Here's how the part is built. I have some questions about the finished solid (model axes, mm). Face numbers are marked on the shaded views. A direction names the side the tool comes from. Coordinates: 2 decimals unless noted, no trailing zeros. Write each loop counter-clockwise with the first axis right and the second up, starting at its lowest first coordinate (ties: lowest second). Pieces come first, ordered by that corner, then holes.
Item 1: If we section it at C-C (x = -3): Please give me the cut outline in (y, z).
Item 2: If we section it at A-A (z = 31.2): Please give me the cut outline in (x, y), then the cut area to 3 significant figures.
Item 3: If I drill on line 1 (X direction, y = 4, z = 31.2); line 2 (X direction, y = 5.75, z = 21), over which ranges is the centre line in solid material (lowest first)?
Item 4: For the marked faces 5 and 6, which set-ups out of +Z, -Z, +X, -X, +Y, -Y let a thin tool reach every point of the face, with its end or its side?
Item 5: If we section it at D-D (y = 8): Please give me the cut outline in (x, z).
Item 6: We'd pull the mould along X, two halves only. Please class the marked faces 1, 2, 3 and 4: +X half, -X half, draft (parallel to the pull), parting line (faces both ways), or undercut.
Item 7: If we section it at B-B (z = -14): Please give me the cut outline in (x, y), then the cut area to 3 significant figures.
Autodesk Inventor part; units mm, degrees
ref_plane "YZ Plane" through (0, 0, 0) normal (1, 0, 0) x (0, 1, 0)
ref_plane "XZ Plane" through (0, 0, 0) normal (0, 1, 0) x (-1, 0, 0)
ref_plane "XY Plane" through (0, 0, 0) normal (0, 0, 1) x (1, 0, 0)
sketch "Boceto1" plane through (0, 0, 0) normal (0, 1, 0) x (-1, 0, 0)
  line L0 (-41.2, 41.2) -> (41.2, 41.2)
  line L1 (41.2, 41.2) -> (41.2, -41.2)
  line L2 (41.2, -41.2) -> (-41.2, -41.2)
  line L3 (-41.2, -41.2) -> (-41.2, 41.2)
  line L4 (-41.2, 41.2) -> (41.2, -41.2) construction
  line L5 (41.2, 41.2) -> (-41.2, -41.2) construction
  line L6 (-21.2, 21.2) -> (21.2, 21.2)
  line L7 (21.2, 21.2) -> (21.2, -21.2)
  line L8 (21.2, -21.2) -> (-21.2, -21.2)
  line L9 (-21.2, -21.2) -> (-21.2, 21.2)
  line L10 (-21.2, 21.2) -> (21.2, -21.2) construction
  line L11 (21.2, 21.2) -> (-21.2, -21.2) construction
  point P0 (0, 0)
  dimension "d0" = 82.4
  dimension "d1" = 82.4
  dimension "d2" = 42.4
  dimension "d3" = 42.4
extrude "Extrusión1" add sketch "Boceto1" along normal blind 15.5
sketch "Boceto2" plane through (0, 15.5, 0) normal (0, 1, 0) x (1, 0, 0)
  circle A0 centre (-31.2, -31.2) radius 2.7
  line L0 (-41.2, 41.2) -> (-41.2, -41.2)
  line L1 (-41.2, -41.2) -> (41.2, -41.2)
  point P0 (0, 0)
  dimension "d6" = 10
  dimension "d7" = 10
  dimension "d8" = 5.4
extrude "Extrusión2" cut sketch "Boceto2" against normal through all
fillet "Empalme1" radius 5 1 edges at (-41.2, 7.75, 41.2)
pattern_circular "Patrón circular1" count 4 over 360 about axis through (0, -10, 0) along (0, 1, 0) of "Extrusión2", "Empalme1"
properties part number "ExtraBase"
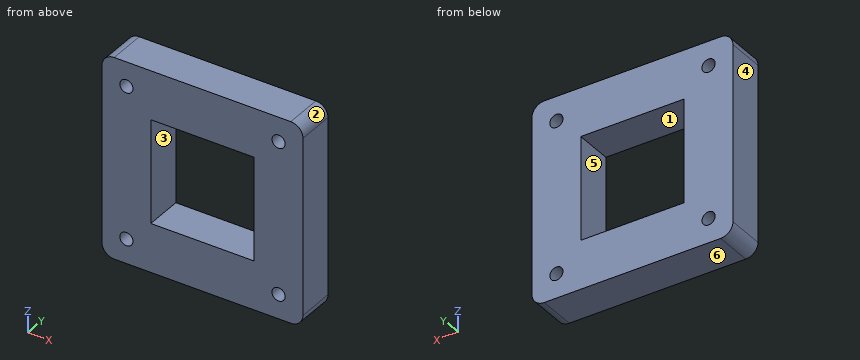
Answer list:
1. outline: (0, -41.2) - (15.5, -41.2) - (15.5, -21.2) - (0, -21.2) - close; (0, 21.2) - (15.5, 21.2) - (15.5, 41.2) - (0, 41.2) - close
2. outline: (-41.2, 0) - (-33.9, 0) - (-33.9, 15.5) - (-41.2, 15.5) - close; (-28.5, 0) - (28.5, 0) - (28.5, 15.5) - (-28.5, 15.5) - close; (33.9, 0) - (41.2, 0) - (41.2, 15.5) - (33.9, 15.5) - close
2. area: 1,110 mm2
3. line 1: x = -41.2 to -33.9, -28.5 to 28.5, 33.9 to 41.2
3. line 2: x = -41.2 to -21.2, 21.2 to 41.2
4. face 5: +Y, -Y
4. face 6: -Z, +X, -X, +Y, -Y
5. outline: (-41.2, -36.2) arc R5 ccw to (-36.2, -41.2) - (36.2, -41.2) arc R5 ccw to (41.2, -36.2) - (41.2, 36.2) arc R5 ccw to (36.2, 41.2) - (-36.2, 41.2) arc R5 ccw to (-41.2, 36.2) - close; hole circle Ø5.4 at (-31.2, -31.2); hole circle Ø5.4 at (-31.2, 31.2); hole (-21.2, -21.2) - (21.2, -21.2) - (21.2, 21.2) - (-21.2, 21.2) - close; hole circle Ø5.4 at (31.2, -31.2); hole circle Ø5.4 at (31.2, 31.2)
6. face 1: undercut
6. face 2: +X half
6. face 3: undercut
6. face 4: -X half
7. outline: (-41.2, 0) - (-21.2, 0) - (-21.2, 15.5) - (-41.2, 15.5) - close; (21.2, 0) - (41.2, 0) - (41.2, 15.5) - (21.2, 15.5) - close
7. area: 620 mm2
